```python
from build123d import *

# Parameters (mm, degrees)
SKETCH1_R           = 127
BOSS_EXTRUDE1_DEPTH = 246.38
FILLET1_R           = 38.1
CHAMFER1_SIZE       = 33.02
CHAMFER1_SIZE2      = 50.846341105
FILLET2_R           = 12.7


with BuildPart() as part:
    # Sketch1 → Boss-Extrude1 (new body)
    with BuildSketch(Plane(origin=(0, 0, 0), x_dir=(1, 0, 0), z_dir=(0, 1, 0))):
        with Locations(Location((0, 0, 0), (0, 0, 90))):
            Circle(SKETCH1_R)
    extrude(amount=BOSS_EXTRUDE1_DEPTH)

    # Fillet1
    fillet1_edges = [part.edges().sort_by_distance(p)[0] for p in [
        (0, 246.38, 127),
    ]]
    fillet(fillet1_edges, radius=FILLET1_R)

    # Chamfer1
    chamfer1_edges = [part.edges().sort_by_distance(p)[0] for p in [
        (0, 0, 127),
    ]]
    chamfer1_side = [part.faces().sort_by_distance(p)[0] for p in [
        (0, 0, 0),
    ]]
    chamfer(chamfer1_edges, length=CHAMFER1_SIZE, length2=CHAMFER1_SIZE2, reference=chamfer1_side[0])

    # Fillet2
    fillet2_edges = [part.edges().sort_by_distance(p)[0] for p in [
        (0, 50.846341105, 127),
    ]]
    fillet(fillet2_edges, radius=FILLET2_R)


solid = part.part
```
Part model, mm, in its own coordinate system. Give positions to 0.01 mm unless a question says otherwise; leave off trailing zeros. Write each loop counter-clockwise with the first axis right and the second up, starting at its lowest first coordinate (ties: lowest second). Pieces come first, ordered by that corner, then holes. Notation, with made-up numbers: (-20.5, 63) -> (-15.5, 63) arc R16 cw to (-15.5, 84) -> close; hole circle Ø8 at (-13.5, 30). An arc over 180 degrees is marked (long way). Put each result on its own line as item: value. Start each with the question number.
Item 1: Cut at B-B (y = 230.5). List the corners of the cut face in (x, z).
Item 2: Wall check: L1, parallel to X at y = 109.5, z = 23; L2, parallel to Z at x = 27, y = 208.5; L3, parallel to Z at x = -116, y = 178.5. Give the ranges that are in metal, low to high. Write a range as [from, to].
Item 3: Pin check, flat tips, straight feed: pin 1 Ø1 at (x, y) = (62.5, 54.5) entering from -Z; pin 2 Ø10 at (x, y) = (97, 148) entering from -Z; pin 3 Ø2 at (x, y) = (-9.5, 154) entering from -Z. Stop position of each tip, or through.
Item 4: Cut at A-A (y = 128). List the corners of the cut face in (x, z), then the cut area to 3 significant figures.
Answer list:
1. outline: circle Ø239.7 at (0, 0)
2. L1: x = [-124.9, 124.9]
2. L2: z = [-124.1, 124.1]
2. L3: z = [-51.7, 51.7]
3. pin 1: stops at z = -110.84
3. pin 2: stops at z = -87.55
3. pin 3: stops at z = -126.72
4. outline: circle Ø254 at (0, 0)
4. area: 50,700 mm2
